Geometry: final body of the model. Coordinates: model frame, mm. A direction names the side the tool comes from. Coordinates: 2 decimals unless noted, no trailing zeros. Write each loop counter-clockwise with the first axis right and the second up, starting at its lowest first coordinate (ties: lowest second). Pieces come first, ordered by that corner, then holes. Notation, with made-up numbers: (4, 68.25) - (9, 68.25) arc R26 ccw to (9, 100.25) - close; hole circle Ø2 at (76, 6). An arc over 180 degrees is marked (long way). Answer as a JSON object with one key per item and string values. Group by question number.
Item 1: Set-up query: faces 4 (the flat face through (20, 7, 0)), 5 (the flat face through (300, 0, 0)), 6 (the flat face through (180, -2, 5)). Return all of +Z, -Z, +X, -X, +Y, -Y with unobstructed straight access to the full face (end or side cutting, diameter ignored); none if empty.
Item 2: Line query: line 1 along X through (y, z) = (-7, -4.25); line 2 along Z through (x, y) = (232, 0.25); line 3 along Y through (x, z) = (259, 4.5). Output: solid intervals per line, ascending. Write a range as from..to.
Item 3: Section A-A on y = 0. Return loops of the section in (x, z), and give its area (3 significant figures).
Item 4: First-contact query: pin 1 Ø2 at (x, y) = (145.5, -2.5) entering from +Z; pin 2 Ø1.8 at (x, z) = (291.5, 1) entering from +Y; pin 3 Ø1.5 at (x, z) = (237, -6.5) entering from -Y; pin 4 Ø12 at (x, z) = (231, 5) entering from -Y. Flat tips, straight axial feed; report the tip coordinate or a pass-through.
Item 5: Mould query, pull axis Z, two halves, no side actions, for faces 1 (the flat face through (289, 2.67, 0)), 2 (the cylindrical face through (239.16, -4.88, 1.08)), 3 (the flat face through (0, 0, 0)). Classes: pulls with the +Z half, pulls with the -Z half, needs draft (parallel to the pull), parting line crosses it, or undercut.
```python
from build123d import *

# Parameters (mm, degrees)
SKETCH_1_R          = 10
EXTRUDE_1_DEPTH     = 150
CUT_EXTRUDE_1_DEPTH = 3
CHAMFER_1_SIZE      = 1
SKETCH_3_R          = 10
EXTRUDE_2_DEPTH     = 150
CUT_EXTRUDE_2_DEPTH = 3
CHAMFER_2_SIZE      = 1
CUT_EXTRUDE_START   = -120
SKETCH_5_R          = 10
SKETCH_5_R_2        = 5
CUT_EXTRUDE_3_DEPTH = 120
SKETCH_6_W          = 6
SKETCH_6_H          = 4.078010131
CUT_EXTRUDE_4_DEPTH = 23


with BuildPart() as part:
    # 草图1 → 凸台-拉伸1 (new body)
    with BuildSketch(Plane(origin=(0, 0, 0), x_dir=(0, 0, -1), z_dir=(1, 0, 0))):
        Circle(SKETCH_1_R)
    extrude(amount=EXTRUDE_1_DEPTH)

    # 草图2 → 切除-拉伸1 (cut)
    with BuildSketch(Plane(origin=(0, 10, 0), x_dir=(1, 0, 0), z_dir=(0, 1, 0))):
        with BuildLine():
            Line((13, 3), (27, 3))
            ThreePointArc((27, 3), (30, 0), (27, -3))
            Line((27, -3), (13, -3))
            ThreePointArc((13, -3), (10, 0), (13, 3))
        make_face()
    extrude(amount=-CUT_EXTRUDE_1_DEPTH, mode=Mode.SUBTRACT)

    # 倒角1
    chamfer_1_edges = [part.edges().sort_by_distance(p)[0] for p in [
        (0, 0, 10),
    ]]
    chamfer(chamfer_1_edges, length=CHAMFER_1_SIZE)

    # 草图3 → 凸台-拉伸2 (add)
    with BuildSketch(Plane(origin=(150, 0, 0), x_dir=(0, 0, -1), z_dir=(1, 0, 0))):
        Circle(SKETCH_3_R)
    extrude(amount=EXTRUDE_2_DEPTH)

    # 草图4 → 切除-拉伸2 (cut)
    with BuildSketch(Plane(origin=(0, 10, 0), x_dir=(1, 0, 0), z_dir=(0, 1, 0))):
        with BuildLine():
            Line((273, 3), (287, 3))
            ThreePointArc((287, 3), (290, 0), (287, -3))
            Line((287, -3), (273, -3))
            ThreePointArc((273, -3), (270, 0), (273, 3))
        make_face()
    extrude(amount=-CUT_EXTRUDE_2_DEPTH, mode=Mode.SUBTRACT)

    # 倒角2
    chamfer_2_edges = [part.edges().sort_by_distance(p)[0] for p in [
        (300, 0, 10),
    ]]
    chamfer(chamfer_2_edges, length=CHAMFER_2_SIZE)

    # 草图5 → 切除-拉伸3 (cut)
    with BuildSketch(Plane(origin=(300, 0, 0), x_dir=(0, 0, -1), z_dir=(1, 0, 0)).offset(CUT_EXTRUDE_START)):
        Circle(SKETCH_5_R)
        Circle(SKETCH_5_R_2, mode=Mode.SUBTRACT)
    extrude(amount=CUT_EXTRUDE_3_DEPTH, mode=Mode.SUBTRACT)

    # 草图6 → 切除-拉伸4 (cut)
    with BuildSketch(Plane(origin=(300, 0, 0), x_dir=(0, 0, -1), z_dir=(1, 0, 0))):
        with Locations((0, 4.709450104)):
            Rectangle(SKETCH_6_W, SKETCH_6_H)
    extrude(amount=-CUT_EXTRUDE_4_DEPTH, mode=Mode.SUBTRACT)


solid = part.part
```
Checks:
{
 "1": {"face 4": "+Y", "face 5": "+Z, -Z, +X, +Y, -Y", "face 6": "+X"},
 "2": {"line 1": "0..180", "line 2": "-4.99..4.99", "line 3": "-2.18..2.18"},
 "3": {"outline": "(0, -9) - (1, -10) - (180, -10) - (180, -5) - (300, -5) - (300, 5) - (180, 5) - (180, 10) - (1, 10) - (0, 9) - close", "area": "4,800 mm^2"},
 "4": {"pin 1": "z = 9.89", "pin 2": "y = 2.67", "pin 3": "through", "pin 4": "y = -5"},
 "5": {"face 1": "undercut", "face 2": "parting line crosses it", "face 3": "needs draft"}
}
